Autodesk Inventor part; units mm, degrees
ref_plane "YZ Plane" through (0, 0, 0) normal (1, 0, 0) x (0, 1, 0)
ref_plane "XZ Plane" through (0, 0, 0) normal (0, 1, 0) x (-1, 0, 0)
ref_plane "XY Plane" through (0, 0, 0) normal (0, 0, 1) x (1, 0, 0)
sketch "Sketch1" plane through (0, 0, 0) normal (0, 1, 0) x (-1, 0, 0)
  line L0 (14.5, -14.5) -> (-14.5, -14.5)
  line L1 (-14.5, -14.5) -> (-14.5, 14.5)
  line L2 (-14.5, 14.5) -> (14.5, 14.5)
  line L3 (14.5, 14.5) -> (14.5, -14.5)
  circle A0 centre (0, 0) radius 4
  dimension "d11" = 29
  dimension "d14" = 29
  dimension "d31" = 8
extrude "Extrusion1" add sketch "Sketch1" along normal blind 10.5 contours A0
sketch "Sketch2" plane through (0, 10.5, 0) normal (0, 1, 0) x (1, 0, 0)
  line L0 (-4.7, 4.7) -> (4.7, 4.7)
  line L1 (4.7, 4.7) -> (4.7, -4.7)
  line L2 (4.7, -4.7) -> (-4.7, -4.7)
  line L3 (-4.7, -4.7) -> (-4.7, 4.7)
  line L4 (14.5, 14.5) -> (-14.5, 14.5)
  line L5 (14.5, -14.5) -> (14.5, 14.5)
  line L6 (-14.5, -14.5) -> (14.5, -14.5)
  line L7 (-14.5, 14.5) -> (-14.5, -14.5)
  point P0 (0, 0)
  dimension "d15" = 9.8
  dimension "d16" = 9.8
  dimension "d17" = 9.8
  dimension "d18" = 9.8
  dimension "d32" = 9.4
  dimension "d50" = 29
extrude "Extrusion2" add sketch "Sketch2" along normal blind 11 contours L0 L1 L2 L3
sketch "Sketch3" plane through (0, 0, 0) normal (0, -1, 0) x (1, 0, 0)
  line L0 (-0.0005, -0.0003) -> (-0.0005, -1.7003)
  line L1 (-0.0005, -1.7003) -> (2.6995, -1.7003)
  line L2 (2.6995, -1.7003) -> (2.6995, 1.6997)
  line L3 (2.6995, 1.6997) -> (-2.7005, 1.6997)
  line L4 (-2.7005, 1.6997) -> (-2.7005, -1.7003)
  line L5 (-2.7005, -1.7003) -> (-0.0005, -1.7003)
  dimension "d42" = 1.7
  dimension "d43" = 2.7
  dimension "d44" = 3.4
  dimension "d45" = 5.4
extrude "Extrusion3" cut sketch "Sketch3" against normal blind 8.2
sketch "Sketch5" plane through (0, 0, 0) normal (0, -1, 0) x (1, 0, 0)
  circle A0 centre (0, 0) radius 2.7
  dimension "d35" = 5.4
extrude "Extrusion4" cut sketch "Sketch5" against normal blind 2.2
fillet "Fillet1" radius 0.635 4 edges at (2.6995, 4.1, 1.6997) (2.6995, 4.1, -1.7003) (-2.7005, 4.1, -1.7003) (-2.7005, 4.1, 1.6997)
equation "\"d14\" = d11"
equation "\"d16\" = d15"
equation "\"d17\" = d15"
equation "\"d18\" = d15"
equation "\"d42\" = 0.5 * d44"
properties part number "Motor_Key_Bearing_2_2"
The listing builds one solid part. Answer for the finished solid, in the listing's coordinates (mm). A direction names the side the tool comes from. Coordinates: 2 decimals unless noted, no trailing zeros. Write each loop counter-clockwise with the first axis right and the second up, starting at its lowest first coordinate (ties: lowest second). Pieces come first, ordered by that corner, then holes. Notation, with made-up numbers: (-4, 76) -> (3, 76) arc R14 ccw to (3, 99) -> close; hole circle Ø1 at (33, 0.25). An arc over 180 degrees is marked (long way). Write each question's results on one line, items separated by ' | '. Start each with the question number.
1) A cutting plane is placed at A-A (y = 5). Determine the outline of the cut face in (x, z) (1 decimal), then the cut area to 3 significant figures.
2) A cutting plane is placed at D-D (y = 8.5). Determine the outline of the cut face in (x, z), then the cut area to 3 significant figures.
3) A tool of negligible diameter and unlimited length cuts with its end or side. For faces 1 (the cylindrical face through (0, 1.1, 2.7)), 2 (the flat face through (0, 16, 4.7)), from which of +Z, -Z, +X, -X, +Y, -Y can it reach the whole face along a straight path? Write none if from no direction.
4) Straight lines are drawn through the part: probe 1 along Y at (x, z) = (-0.25, -0.5); probe 2 along Y at (x, z) = (2, -3.5); probe 3 along X at (y, z) = (5.5, 1.5). For each, find the intervals that lie inside material, in ascending order.
5) For a pull along X with two mould halves and no side action, classify faces 3 (the flat face through (4.7, 16, 0)), 4 (the flat face through (0, 5, -1.7)), 5 (the flat face through (-4.7, 16, 0)) as +X half, -X half, draft (parallel to the pull), parting line (faces both ways), or undercut.
6) A cutting plane is placed at C-C (x = 0). Determine the outline of the cut face in (y, z).
7) A cutting plane is placed at B-B (z = -3.75). Determine the outline of the cut face in (x, y).
8) Flat-ended cylindrical pins translate along their axes: pin 1 Ø4.5 at (x, y) = (0.5, 5.5) entering from +Z; pin 2 Ø3.5 at (x, y) = (-0.5, 6.5) entering from -Z; pin 3 Ø2.5 at (y, z) = (2.5, 0) entering from -X. Find the tip coordinate at first contact, or state that the pin passes through.
Values follow:
1) outline: circle Ø8 at (0, 0); hole (-2.7, -1.1) arc R0.6 ccw to (-2.1, -1.7) -> (2.1, -1.7) arc R0.6 ccw to (2.7, -1.1) -> (2.7, 1.1) arc R0.6 ccw to (2.1, 1.7) -> (-2.1, 1.7) arc R0.6 ccw to (-2.7, 1.1) -> close | area: 32.3 mm²
2) outline: circle Ø8 at (0, 0) | area: 50.3 mm²
3) face 1: -Y | face 2: +Z, +X, -X, +Y, -Y
4) probe 1: 8.2 to 21.5 | probe 2: 10.5 to 21.5 | probe 3: -3.71 to -2.53, 2.53 to 3.71
5) face 3: +X half | face 4: undercut | face 5: -X half
6) outline: (0, -4) -> (10.5, -4) -> (10.5, -4.7) -> (21.5, -4.7) -> (21.5, 4.7) -> (10.5, 4.7) -> (10.5, 4) -> (0, 4) -> (0, 2.7) -> (2.2, 2.7) -> (2.2, 1.7) -> (8.2, 1.7) -> (8.2, -1.7) -> (2.2, -1.7) -> (2.2, -2.7) -> (0, -2.7) -> close
7) outline: (-4.7, 10.5) -> (-1.39, 10.5) -> (-1.39, 0) -> (1.39, 0) -> (1.39, 10.5) -> (4.7, 10.5) -> (4.7, 21.5) -> (-4.7, 21.5) -> close
8) pin 1: z = 4 | pin 2: z = -4 | pin 3: x = -4
